Part model, mm, in its own coordinate system. Face numbers are marked on the shaded views. Coordinates: 2 decimals unless noted, no trailing zeros. Use a Markdown table: item, result. Add a question column.
Q1. Mould opens along Z. For the marked faces 1 and 2 say: released by +Z, released by -Z, zero draft, split by the parting line, or undercut.
Q2. Pin check, flat tips, straight feed: pin 1 Ø1 at (y, z) = (-3.5, 11.5) entering from +X; pin 2 Ø1.2 at (y, z) = (-3, 0.5) entering from -X; pin 3 Ø3 at (x, y) = (-12, -3.5) entering from -Z. Stop position of each tip, or through.
Q3. Wall check: L1, parallel to Z at x = -1, y = -3.7; L2, parallel to Z at x = 13.5, y = -0.4; L3, parallel to Z at x = -0.5, y = -2.5. Give the ranges that are in metal, low to high. Write a range as from..to.
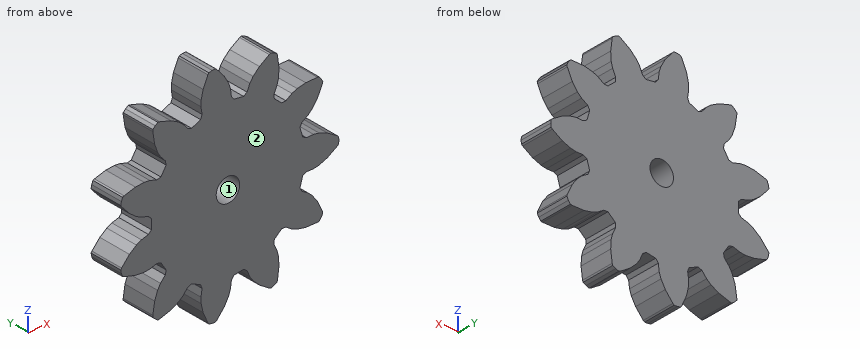
from build123d import *

# Parameters (mm, degrees)
F1_DEPTH = 5
F2_R     = 1.75
F3_DEPTH = 25


with BuildPart() as f1:
    # F0 (on Front) → F1 (new body)
    with BuildSketch(Plane.XZ):
        Polygon((-15.759088, 5.238458), (-15.984615, 5.125695), (-16.169742, 4.663269), (-16.264009, 4.174165), (-16.135249, 3.957374), (-14.96593, 2.641114), (-13.930142, 1.847068), (-13.170214, 1.467105), (-12.134025, 1.176704), (-11.697261, 0.730628), (-11.697261, -0.730628), (-12.134025, -1.176704), (-13.170214, -1.467105), (-13.930142, -1.847068), (-14.96593, -2.641114), (-16.135249, -3.957374), (-16.264009, -4.174165), (-16.169742, -4.663269), (-15.984615, -5.125695), (-15.759088, -5.238458), (-14.063771, -5.713585), (-12.763117, -5.821589), (-11.918401, -5.730387), (-10.889701, -5.414481), (-10.281105, -5.553612), (-9.49109, -6.782899), (-9.617352, -7.394294), (-10.332048, -8.198801), (-10.765916, -8.929295), (-11.207983, -10.157278), (-11.480053, -11.896767), (-11.471167, -12.148757), (-11.127434, -12.509253), (-10.721689, -12.798183), (-10.471, -12.771117), (-8.787936, -12.254261), (-7.635364, -11.641933), (-6.974052, -11.108521), (-6.279446, -10.286607), (-5.692242, -10.074619), (-4.363037, -10.681647), (-4.13871, -11.264248), (-4.305001, -12.327436), (-4.275059, -13.176533), (-3.983052, -14.448578), (-3.271493, -16.059021), (-3.127781, -16.266204), (-2.643716, -16.383637), (-2.146174, -16.407338), (-1.949914, -16.249036), (-0.813464, -14.904296), (-0.174908, -13.766046), (0.093039, -12.959779), (0.233018, -11.892808), (0.612396, -11.397006), (2.058779, -11.189048), (2.562472, -11.557883), (2.997382, -12.542197), (3.481627, -13.240315), (4.414999, -14.152556), (5.884272, -15.12265), (6.117181, -15.219247), (6.587892, -15.056333), (7.019264, -14.80728), (7.098784, -14.568001), (7.327805, -12.822322), (7.249608, -11.519536), (7.039119, -10.696398), (6.580029, -9.723126), (6.631132, -9.100924), (7.735475, -8.144005), (8.358617, -8.181972), (9.256646, -8.774899), (10.041451, -9.100391), (11.319848, -9.363198), (13.080351, -9.384944), (13.328511, -9.340286), (13.63642, -8.948748), (13.864665, -8.506014), (13.802197, -8.261728), (13.051077, -6.669352), (12.280954, -5.615655), (11.658857, -5.036986), (10.746456, -4.466421), (10.453058, -3.915363), (10.864742, -2.513298), (11.409488, -2.208342), (12.48552, -2.221633), (13.321713, -2.071157), (14.539253, -1.60109), (16.032039, -0.667584), (16.216661, -0.495851), (16.264009, 0), (16.216661, 0.495851), (16.032039, 0.667584), (14.539253, 1.60109), (13.321713, 2.071157), (12.48552, 2.221633), (11.409488, 2.208342), (10.864742, 2.513298), (10.453058, 3.915363), (10.746456, 4.466421), (11.658857, 5.036986), (12.280954, 5.615655), (13.051077, 6.669352), (13.802197, 8.261728), (13.864665, 8.506014), (13.63642, 8.948748), (13.328511, 9.340286), (13.080351, 9.384944), (11.319848, 9.363198), (10.041451, 9.100391), (9.256646, 8.774899), (8.358617, 8.181972), (7.735475, 8.144005), (6.631132, 9.100924), (6.580029, 9.723126), (7.039119, 10.696398), (7.249608, 11.519536), (7.327805, 12.822322), (7.098784, 14.568001), (7.019264, 14.80728), (6.587892, 15.056333), (6.117181, 15.219247), (5.884272, 15.12265), (4.414999, 14.152556), (3.481627, 13.240315), (2.997382, 12.542197), (2.562472, 11.557883), (2.058779, 11.189048), (0.612396, 11.397006), (0.233018, 11.892808), (0.093039, 12.959779), (-0.174908, 13.766046), (-0.813464, 14.904296), (-1.949914, 16.249036), (-2.146174, 16.407338), (-2.643716, 16.383637), (-3.127781, 16.266204), (-3.271493, 16.059021), (-3.983052, 14.448578), (-4.275059, 13.176533), (-4.305001, 12.327436), (-4.13871, 11.264248), (-4.363037, 10.681647), (-5.692242, 10.074619), (-6.279446, 10.286607), (-6.974052, 11.108521), (-7.635364, 11.641933), (-8.787936, 12.254261), (-10.471, 12.771117), (-10.721689, 12.798183), (-11.127434, 12.509253), (-11.471167, 12.148757), (-11.480053, 11.896767), (-11.207983, 10.157278), (-10.765916, 8.929295), (-10.332048, 8.198801), (-9.617352, 7.394294), (-9.49109, 6.782899), (-10.281105, 5.553612), (-10.889701, 5.414481), (-11.918401, 5.730387), (-12.763117, 5.821589), (-14.063771, 5.713585), align=None)
        Polygon((-1.27575, 1.161973), (-1.01258, 1.341924), (-0.717747, 1.463227), (-0.404136, 1.520579), (-0.085455, 1.511475), (0.22437, 1.436313), (0.511798, 1.298376), (0.764266, 1.103694), (0.97074, 0.860776), (1.122196, 0.580237), (1.212016, 0.27434), (1.236273, -0.043548), (1.193908, -0.359532), (1.086771, -0.659803), (0.919546, -0.931238), (0.699541, -1.161973), (0.436371, -1.341924), (0.141537, -1.463227), (-0.172073, -1.520579), (-0.490755, -1.511475), (-0.80058, -1.436313), (-1.088008, -1.298376), (-1.340475, -1.103694), (-1.546949, -0.860776), (-1.698406, -0.580237), (-1.788226, -0.27434), (-1.812483, 0.043548), (-1.770117, 0.359532), (-1.662981, 0.659803), (-1.495756, 0.931238), align=None, mode=Mode.SUBTRACT)
    extrude(amount=F1_DEPTH)

    # F2 (on face) → F3 (cut)
    with BuildSketch(Plane.XZ.offset(5)):
        with Locations((-0.282437, 0)):
            Circle(F2_R)
    extrude(amount=-F3_DEPTH, mode=Mode.SUBTRACT)


solid = f1.part
Recorded:
| question | item | result |
|---|---|---|
| 1 | face 1 | undercut |
| 1 | face 2 | zero draft |
| 2 | pin 1 | x = 7.28 |
| 2 | pin 2 | x = -12.06 |
| 2 | pin 3 | z = -12.8 |
| 3 | L1 | -15.13..-1.6, 1.6..15.13 |
| 3 | L2 | -9.12..-7.62, -2..2, 7.62..9.12 |
| 3 | L3 | -14.35..-1.74, 1.74..14.35 |
